```python
from build123d import *


with BuildPart() as f1:
    # F0 (on Front) → F1 (revolve)
    with BuildSketch(Plane.XZ):
        Polygon((-21.084563, 49.019749), (-24.64242, 55.369749), (-41.635697, 27.61407), (-22.981961, 16.193413), (-29.173962, -6.938921), (0, -6.089257), (0, 13.73623), (0, 21.609018), (-5.112027, 21.609018), (-19.666283, 21.609018), (-32.904414, 29.713998), align=None)
        with BuildLine():
            Line((-5.112027, 32.483828), (-5.112027, 21.609018))
            Line((-5.112027, 21.609018), (0, 21.609018))
            Line((0, 21.609018), (0, 30.065285))
            ThreePointArc((0, 30.065285), (-2.827639, 30.700427), (-5.112027, 32.483828))
        make_face()
        with BuildLine():
            ThreePointArc((0, 43.289019), (-5.976725, 39.504791), (-5.112027, 32.483828))
            ThreePointArc((-5.112027, 32.483828), (-2.827639, 30.700427), (0, 30.065285))
            Line((0, 30.065285), (0, 43.289019))
        make_face()
        Polygon((0, -6.089257), (-29.173962, -6.938921), (-41.918916, -17.984549), (-39.653149, -34.12816), (0, -34.12816), (0, -18.245815), align=None)
    revolve(axis=Axis((0, 0, 3.823487), (0, 0, -1)))


solid = f1.part
```
Geometry: final body of the model. Coordinates: model frame, mm. A direction names the side the tool comes from. Coordinates: 2 decimals unless noted, no trailing zeros. Loops run counter-clockwise (first coordinate to the right, second up) from the corner with the lowest first, then second, coordinate; pieces in that order, holes last. Notation, with made-up numbers: (-20.75, 35.25) -> (12.25, 35.25) arc R22 ccw to (12.25, 71.25) -> close; hole circle Ø10 at (2.5, -12). An arc over 180 degrees is marked (long way). Use a Markdown table: item, result. Add a question column.
(1) Line query: line 1 along Z through (x, y) = (15.5, 26.5); line 2 along Z through (x, y) = (37, 9.5); line 3 along Y through (x, z) = (1.5, 29.5). Output: solid intervals per line, ascending.
(2) Access query for faces 5 (the conical face through (5.572, -25.094, 53.633)), 6 (the cylindrical face through (4.057, -3.111, 26.97)). Directions: +Z, -Z, +X, -X, +Y, -Y. A direction counts if a zero-diameter tool reaches every point of the face in a straight line with its end or side. Return the directions, or none.
(3) Pin query (flat end, axial travel): pin 1 Ø2 at (x, z) = (-9, 2) entering from -Y; pin 2 Ø12 at (x, y) = (5, -8.5) entering from +Z; pin 3 Ø1.5 at (y, z) = (8, -8) entering from -X. Return the tip coordinate at first contact, or that it passes through.
(4) Section query A-A, the plane z = -21. Return loops of the section in (x, y).
(5) Mould query, pull axis Y, two halves, no side actions, for faces 1 (the conical face through (-22.785, 7.175, 16.748)), 2 (the conical face through (-10, -19.2, 48.1)), 3 (the flat face through (1, 1, -34.128)), 4 (the conical face through (-20.323, 6.4, 49.417)). Classes: pulls with the +Y half, pulls with the -Y half, needs draft (parallel to the pull), parting line crosses it, or undercut.
Answer:
| question | item | result |
|---|---|---|
| 1 | line 1 | z = -34.13 to -8.26, 20.92 to 28.36, 33.31 to 45.48 |
| 1 | line 2 | z = -34.13 to -14.76, 25.51 to 33.23 |
| 1 | line 3 | y = -40.45 to -32.52, -4.89 to 4.89, 32.52 to 40.45 |
| 2 | face 5 | +Z |
| 2 | face 6 | none |
| 3 | pin 1 | stops at y = -25.66 |
| 3 | pin 2 | stops at z = 42.04 |
| 3 | pin 3 | stops at x = -30.24 |
| 4 | outline | circle Ø82.99 at (0, 0) |
| 5 | face 1 | parting line crosses it |
| 5 | face 2 | undercut |
| 5 | face 3 | needs draft |
| 5 | face 4 | undercut |
